Could you check a few things on this model? Use its own coordinates, in mm. A direction names the side the tool comes from. Round coordinates to 2 decimals unless told otherwise and drop trailing zeros. Write each loop counter-clockwise with the first axis right and the second up, starting at its lowest first coordinate (ties: lowest second). Pieces come first, ordered by that corner, then holes. Notation, with made-up numbers: (-12, 58.25) -> (14, 58.25) arc R16 cw to (14, 73.25) -> close; hole circle Ø11 at (84.25, -14.75). An arc over 180 degrees is marked (long way). One line per question, with ' | ' between items. Start each with the question number.
1. Imagine slicing it at A-A, the plane x = 20. List the corners of the cut face in (y, z) for me, and give its area (3 significant figures).
2. Imagine slicing it at C-C, the plane z = -3.25. List the corners of the cut face in (x, y) for me, and give its area (3 significant figures).
3. For pin 1 Ø3 at (y, z) = (2.5, -1) entering from -X; pin 2 Ø3 at (x, z) = (-5, 2.5) entering from +Y, each with a flat end and sliding along its axis, tell me the tip position at first contact or that it passes through.
4. For faces 5 (the flat face through (0, 5, 0)), 6 (the flat face through (65, 10, 0)), 7 (the flat face through (-5, 140, 0)), 8 (the flat face through (29, 76, -5)), 9 (the flat face through (65, 140, 0)), which set-ups out of +Z, -Z, +X, -X, +Y, -Y let a thin tool reach every point of the face, with its end or its side?
5. Imagine slicing it at B-B, the plane y = 112.5. List the corners of the cut face in (x, z) for me.
6. If I drill on line 1 along Y through (x, z) = (20, 1.25); line 2 along X through (y, z) = (37.5, 1.75); line 3 along Y through (x, z) = (27, -0.25), over which ranges is the centre line in solid material (lowest first)? Write a range as [from, to].
7. Thinking about a two-plate mould opening in Y: for faces 1 (the cylindrical face through (24.166, 105.965, -0.07)), 2 (the flat face through (0, 145, 0)), 3 (the flat face through (30, 150, 0)), 4 (the cylindrical face through (24.166, 30.965, -0.07)), which applies, released by +Y, released by -Y, zero draft, split by the parting line, or undercut?
from build123d import *

# Parameters (mm, degrees)
PAD_DEPTH    = 5
SKETCH001_R  = 7.75
POCKET_DEPTH = 10.001


with BuildPart() as part:
    # Sketch → Pad (new body, symmetric)
    with BuildSketch(Plane.XY):
        Polygon((-10, 140), (-10, 10), (0, 10), (0, 0), (60, 0), (60, 10), (70, 10), (70, 140), (60, 140), (60, 150), (0, 150), (0, 140), align=None)
    extrude(amount=PAD_DEPTH, both=True)

    # Sketch001 (on Face13 of Pad) → Pocket (cut, through all)
    with BuildSketch(Plane(origin=(0, 0, -5), x_dir=(1, 0, 0), z_dir=(0, 0, -1))):
        with Locations((20, -37.5)):
            Circle(SKETCH001_R)
        with Locations((20, -112.5)):
            Circle(SKETCH001_R)
    extrude(amount=-POCKET_DEPTH, mode=Mode.SUBTRACT)


solid = part.part
Geometry results:
1) outline: (0, -5) -> (29.75, -5) -> (29.75, 5) -> (0, 5) -> close; (45.25, -5) -> (104.75, -5) -> (104.75, 5) -> (45.25, 5) -> close; (120.25, -5) -> (150, -5) -> (150, 5) -> (120.25, 5) -> close | area: 1,190 mm2
2) outline: (-10, 10) -> (0, 10) -> (0, 0) -> (60, 0) -> (60, 10) -> (70, 10) -> (70, 140) -> (60, 140) -> (60, 150) -> (0, 150) -> (0, 140) -> (-10, 140) -> close; hole circle Ø15.5 at (20, 37.5); hole circle Ø15.5 at (20, 112.5) | area: 11,200 mm2
3) pin 1: stops at x = 0 | pin 2: stops at y = 140
4) face 5: +Z, -Z, -X, -Y | face 6: +Z, -Z, +X, -Y | face 7: +Z, -Z, -X, +Y | face 8: -Z, +X, -X, +Y, -Y | face 9: +Z, -Z, +X, +Y
5) outline: (-10, -5) -> (12.25, -5) -> (12.25, 5) -> (-10, 5) -> close; (27.75, -5) -> (70, -5) -> (70, 5) -> (27.75, 5) -> close
6) line 1: y = [0, 29.75], [45.25, 104.75], [120.25, 150] | line 2: x = [-10, 12.25], [27.75, 70] | line 3: y = [0, 34.17], [40.83, 109.17], [115.83, 150]
7) face 1: undercut | face 2: zero draft | face 3: released by +Y | face 4: undercut
